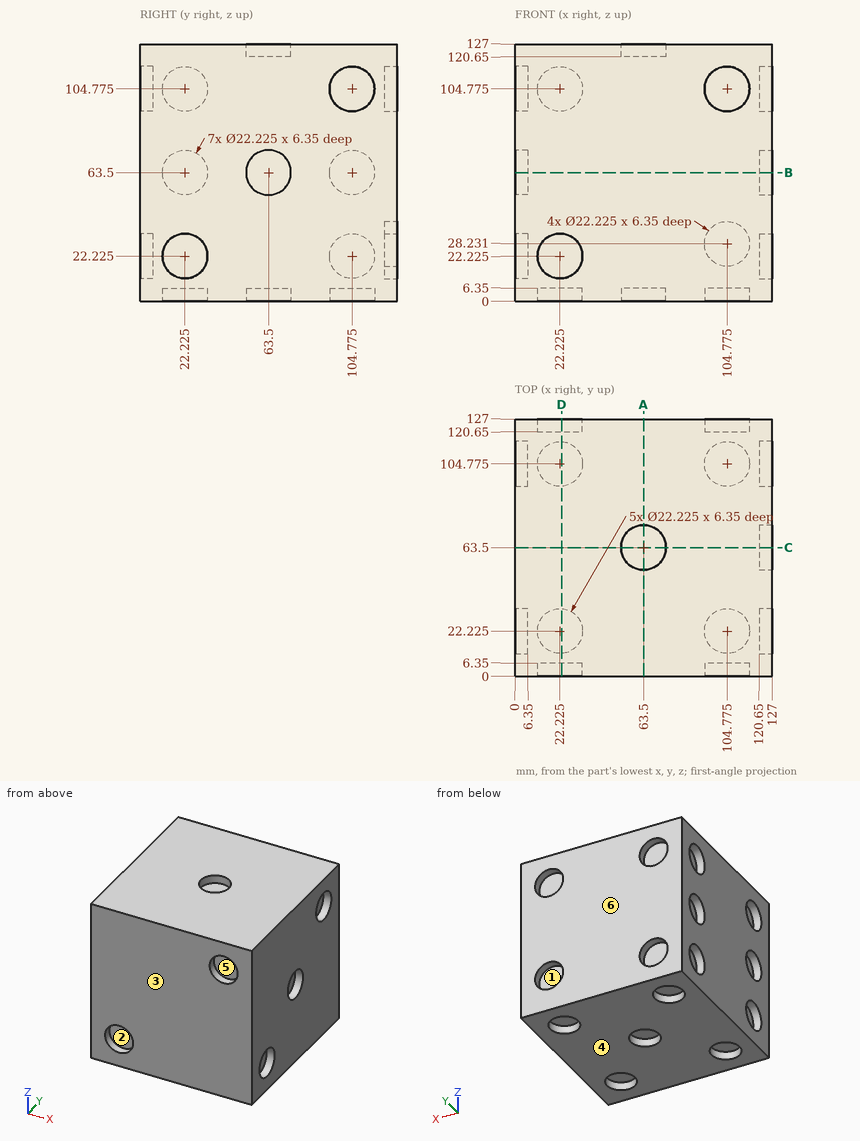
Check sheet for the drawn part. Datum: minimum x, y, z corner. Units: mm. A direction names the side the tool comes from. Round coordinates to 2 decimals unless told otherwise and drop trailing zeros. Loops run counter-clockwise (first coordinate to the right, second up) from the corner with the lowest first, then second, coordinate; pieces in that order, holes last. Notation, with made-up numbers: (41, 75.25) -> (93, 75.25) arc R29 ccw to (93, 109.25) -> close; hole circle Ø1 at (3, -25). An arc over 180 degrees is marked (long way). Put each result on its own line as item: value. Start each with the question number.
1. Section check A-A (x = 63.5). Enter the section's corners in (y, z), plus the area to 3 significant figures.
2. Section check B-B (z = 63.5). Enter the section's corners in (x, y).
3. Section check C-C (y = 63.5). Enter the section's corners in (x, z), plus the area to 3 significant figures.
4. Section check D-D (x = 23). Enter the section's corners in (y, z).
5. Gauge pin test, flat ends, axial feed: pin 1 (20 mm diameter, centred on x = 104.775, y = 104.775, fed in from -Z); pin 2 (20 mm diameter, centred on y = 104.775, z = 104.775, fed in from +X); pin 3 (20 mm diameter, centred on x = 22.225, z = 22.225, fed in from -Y). Record the tip position at first contact, or that the pin passes through.
6. Access from +Z, -Z, +X, -X, +Y, -Y to the whole of each face (thin tool, end or side, straight path). Record for the marked faces 1, 2 and 3.
7. Draft check along Z on the marked faces 4, 5 and 6. Enter one of: +Z half, -Z half, draft (parallel to the pull), parting line (faces both ways), or undercut.
8. Scan lines: probe 1 along Z at (x, y) = (31.5, 106); probe 2 along X at (y, z) = (29.5, 18). Record each from-to range of solid material in increasing order.
Findings:
1. outline: (0, 0) -> (52.39, 0) -> (52.39, 6.35) -> (74.61, 6.35) -> (74.61, 0) -> (127, 0) -> (127, 127) -> (74.61, 127) -> (74.61, 120.65) -> (52.39, 120.65) -> (52.39, 127) -> (0, 127) -> close
1. area: 15,800 mm^2
2. outline: (0, 0) -> (127, 0) -> (127, 52.39) -> (120.65, 52.39) -> (120.65, 74.61) -> (127, 74.61) -> (127, 127) -> (0, 127) -> (0, 115.89) -> (6.35, 115.89) -> (6.35, 93.66) -> (0, 93.66) -> (0, 33.34) -> (6.35, 33.34) -> (6.35, 11.11) -> (0, 11.11) -> close
3. outline: (0, 0) -> (52.39, 0) -> (52.39, 6.35) -> (74.61, 6.35) -> (74.61, 0) -> (127, 0) -> (127, 52.39) -> (120.65, 52.39) -> (120.65, 74.61) -> (127, 74.61) -> (127, 127) -> (74.61, 127) -> (74.61, 120.65) -> (52.39, 120.65) -> (52.39, 127) -> (0, 127) -> close
3. area: 15,700 mm^2
4. outline: (0, 0) -> (11.14, 0) -> (11.14, 6.35) -> (33.31, 6.35) -> (33.31, 0) -> (93.69, 0) -> (93.69, 6.35) -> (115.86, 6.35) -> (115.86, 0) -> (127, 0) -> (127, 11.14) -> (120.65, 11.14) -> (120.65, 33.31) -> (127, 33.31) -> (127, 93.69) -> (120.65, 93.69) -> (120.65, 115.86) -> (127, 115.86) -> (127, 127) -> (0, 127) -> (0, 33.31) -> (6.35, 33.31) -> (6.35, 11.14) -> (0, 11.14) -> close
5. pin 1: stops at z = 6.35
5. pin 2: stops at x = 120.65
5. pin 3: stops at y = 6.35
6. face 1: +Y
6. face 2: -Y
6. face 3: +Z, -Z, +X, -X, -Y
7. face 4: -Z half
7. face 5: undercut
7. face 6: draft
8. probe 1: z = 6.35 to 127
8. probe 2: x = 6.35 to 120.65
